Check sheet for the drawn part. Datum: minimum x, y, z corner. Units: mm. Coordinates: 2 decimals unless noted, no trailing zeros. Write each loop counter-clockwise with the first axis right and the second up, starting at its lowest first coordinate (ties: lowest second). Pieces come first, ordered by that corner, then holes. Notation, with made-up numbers: (89.5, -30) -> (97.5, -30) arc R10 ccw to (97.5, -18) -> close; hole circle Ø3 at (59.5, 45). An arc over 180 degrees is marked (long way). Answer in a Markdown table with one row per item. Add a question column.
1. Cross-section at A-A on x = 24. Record the cut outline in (y, z), and give its area (4 significant figures).
2. Depth check by flat-ended pin: P1, Ø6, axis at x = 24, y = 65, coming from the -Z side; P2, Ø3.5, axis at x = 24, y = 25, coming from the -Z side. Enter the tip coordinate at first touch or a pass-through.
3. Cross-section at C-C on z = 3.5. Record the cut outline in (x, y).
4. Cross-section at D-D on x = 134. Record the cut outline in (y, z).
5. Cross-section at B-B on y = 65. Record the cut outline in (x, z).
6. Scan lines: L1, parallel to Y at x = 24, z = 3.25; L2, parallel to Y at x = 27, z = 4.5; L3, parallel to X at y = 64.5, z = 2. Record each from-to range of solid material in increasing order. Write a range as from..to.
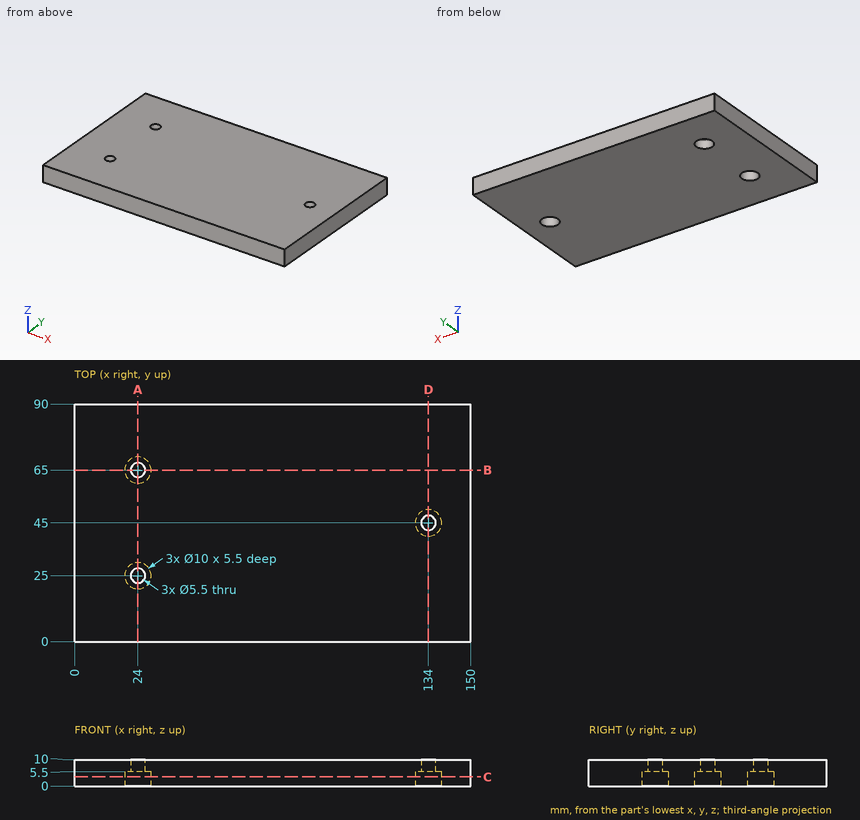
Results found:
| question | item | result |
|---|---|---|
| 1 | outline | (0, 0) -> (20, 0) -> (20, 5.5) -> (22.25, 5.5) -> (22.25, 10) -> (0, 10) -> close; (27.75, 5.5) -> (30, 5.5) -> (30, 0) -> (60, 0) -> (60, 5.5) -> (62.25, 5.5) -> (62.25, 10) -> (27.75, 10) -> close; (67.75, 5.5) -> (70, 5.5) -> (70, 0) -> (90, 0) -> (90, 10) -> (67.75, 10) -> close |
| 1 | area | 740.5 mm^2 |
| 2 | P1 | stops at z = 5.5 |
| 2 | P2 | passes through |
| 3 | outline | (0, 0) -> (150, 0) -> (150, 90) -> (0, 90) -> close; hole circle Ø10 at (24, 25); hole circle Ø10 at (24, 65); hole circle Ø10 at (134, 45) |
| 4 | outline | (0, 0) -> (40, 0) -> (40, 5.5) -> (42.25, 5.5) -> (42.25, 10) -> (0, 10) -> close; (47.75, 5.5) -> (50, 5.5) -> (50, 0) -> (90, 0) -> (90, 10) -> (47.75, 10) -> close |
| 5 | outline | (0, 0) -> (19, 0) -> (19, 5.5) -> (21.25, 5.5) -> (21.25, 10) -> (0, 10) -> close; (26.75, 5.5) -> (29, 5.5) -> (29, 0) -> (150, 0) -> (150, 10) -> (26.75, 10) -> close |
| 6 | L1 | y = 0..20, 30..60, 70..90 |
| 6 | L2 | y = 0..21, 29..61, 69..90 |
| 6 | L3 | x = 0..19.03, 28.97..150 |
